The figure shows three views and two pictorial views of one solid part (mm, origin at its lowest corner). Answer the questions. Round coordinates to 2 decimals unless told otherwise and drop trailing zeros. Order: outer loops, then holes, each group sorted by start corner. A loop starts at its lowest first (then second) coordinate and runs counter-clockwise, first axis right, second up. Notation, with made-up numbers: (-27, 36.25) - (-5, 36.25) arc R19 cw to (-5, 52.25) - close; hole circle Ø3 at (-3, 9). An arc over 180 degrees is marked (long way). Answer as a JSON object with one key per item and string values. Group by question number.
Q1. A cutting plane is placed at A-A on x = 32.5. Determine the outline of the cut face in (y, z).
Q2. A cutting plane is placed at C-C on x = 39. Determine the outline of the cut face in (y, z).
Q3. The mould has two halves that part along Y. Classify the marked faces 1, 2 and 3: pulls with the +Y half, pulls with the -Y half, needs draft (parallel to the pull), parting line crosses it, or undercut.
Q4. Given pin 1 Ø21.5 at (x, y) = (32.5, 32.5) entering from +Z; pin 2 Ø1 at (y, z) = (10, 1) entering from +X; pin 3 Ø1 at (x, z) = (31.5, 3) entering from +Y; pin 4 Ø2 at (y, z) = (41, 0.5) entering from +X, each flat-ended and moving along its own axis, determine where each tip first touches the part or whether it passes through.
Q5. A cutting plane is placed at D-D on z = 2. Determine the outline of the cut face in (x, y).
Q6. A cutting plane is placed at B-B on y = 32.5. Determine the outline of the cut face in (x, z).
Q7. Consider line 1 (Y direction, x = 32.5, z = 1.3); line 2 (Y direction, x = 32, z = 2.35) (1 decimal); line 3 (X direction, y = 23, z = 1.2). Determine where each line is inside the solid, lowest interval first.
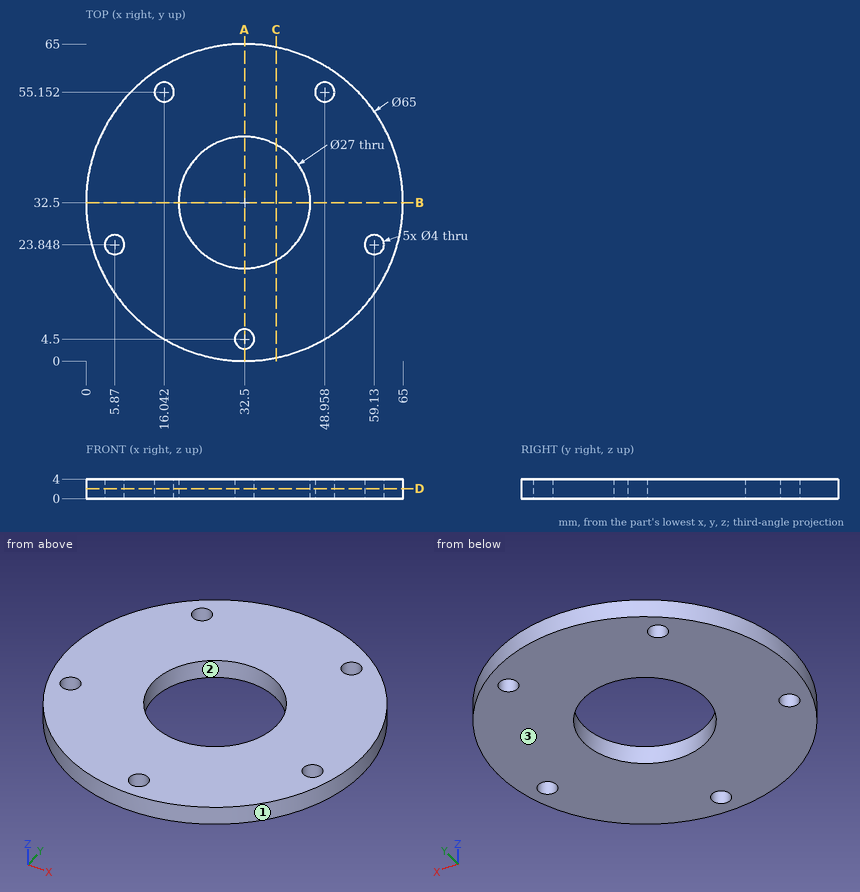
Result set:
{
 "1": {"outline": "(0, 0) - (2.5, 0) - (2.5, 4) - (0, 4) - close; (6.5, 0) - (19, 0) - (19, 4) - (6.5, 4) - close; (46, 0) - (65, 0) - (65, 4) - (46, 4) - close"},
 "2": {"outline": "(0.66, 0) - (20.67, 0) - (20.67, 4) - (0.66, 4) - close; (44.33, 0) - (64.34, 0) - (64.34, 4) - (44.33, 4) - close"},
 "3": {"face 1": "parting line crosses it", "face 2": "undercut", "face 3": "needs draft"},
 "4": {"pin 1": "passes through", "pin 2": "stops at x = 56.42", "pin 3": "stops at y = 65", "pin 4": "stops at x = 64.12"},
 "5": {"outline": "circle Ø65 at (32.5, 32.5); hole circle Ø4 at (5.87, 23.85); hole circle Ø4 at (16.04, 55.15); hole circle Ø27 at (32.5, 32.5); hole circle Ø4 at (32.5, 4.5); hole circle Ø4 at (48.96, 55.15); hole circle Ø4 at (59.13, 23.85)"},
 "6": {"outline": "(0, 0) - (19, 0) - (19, 4) - (0, 4) - close; (46, 0) - (65, 0) - (65, 4) - (46, 4) - close"},
 "7": {"line 1": "y = 0 to 2.5, 6.5 to 19, 46 to 65", "line 2": "y = 0 to 2.6, 6.4 to 19, 46 to 65", "line 3": "x = 1.42 to 4.06, 7.68 to 22.91, 42.09 to 57.32, 60.94 to 63.58"}
}
